Autodesk Inventor part; units mm, degrees
ref_plane "YZ Plane" through (0, 0, 0) normal (1, 0, 0) x (0, 1, 0)
ref_plane "XZ Plane" through (0, 0, 0) normal (0, 1, 0) x (-1, 0, 0)
ref_plane "XY Plane" through (0, 0, 0) normal (0, 0, 1) x (1, 0, 0)
sketch "スケッチ1" plane through (0, 0, 0) normal (0, 1, 0) x (-1, 0, 0)
  line L0 (0, 0) -> (-38, 0)
  line L1 (-38, 0) -> (-38, -48)
  line L2 (-38, -48) -> (0, -48)
  line L3 (0, -48) -> (0, 0)
  dimension "d0" = 48
  dimension "d1" = 38
extrude "押し出し1" add sketch "スケッチ1" along normal blind 46
sketch "スケッチ2" plane through (38, 0, -48) normal (0, 0, -1) x (-1, 0, 0)
  line L0 (3, 43) -> (59.072, 43)
  line L1 (59.072, 43) -> (59.072, 3)
  line L2 (59.072, 3) -> (3, 3)
  line L3 (3, 3) -> (3, 43)
  line L4 (0, 46) -> (38, 46)
  line L5 (0, 0) -> (38, 0)
  line L6 (0, 0) -> (0, 46)
  dimension "d4" = 40
  dimension "d6" = 3
  dimension "d7" = 3
extrude "押し出し2" cut sketch "スケッチ2" against normal blind 100
sketch "スケッチ3" plane through (0, 46, 0) normal (0, 1, 0) x (1, 0, 0)
  line L0 (38, 48) -> (0, 48)
  line L1 (38, 0) -> (38, 48)
  point P0 (0, 0)
  point P1 (17, 32)
  dimension "d10" = 16
  dimension "d11" = 21
hole "穴1" at (17, 46, -32) direction (0, -1, 0) diameter 22 end through all
sketch "スケッチ4" plane through (0, 46, 0) normal (0, 1, 0) x (1, 0, 0)
  line L0 (0, 0) -> (38, 0)
  line L1 (38, 0) -> (38, 48)
  point P0 (30.5, 4)
  point P1 (30.5, 31)
  point P2 (3.5, 4)
  point P3 (3.5, 31)
  point P4 (3.5, 4)
  dimension "d19" = 4
  dimension "d20" = 7.5
  dimension "d23" = 27
  dimension "d26" = 27
hole "穴2" at (30.5, 46, -4) at (30.5, 46, -31) at (3.5, 46, -31) at (3.5, 46, -4) direction (0, -1, 0) diameter 3.2 end through all
sketch "スケッチ6" plane through (38, 0, 0) normal (1, 0, 0) x (0, 0, -1)
  line L0 (0, 46) -> (48, 46)
  line L1 (0, 0) -> (0, 46)
  point P0 (10, 31)
  point P1 (32, 31)
  point P2 (10, 16)
  point P3 (32, 16)
  dimension "d45" = 15
  dimension "d46" = 10
  dimension "d49" = 22
  dimension "d52" = 15
fillet "フィレット1" radius 2 2 edges at (35, 3, -24) (35, 43, -24)
sketch "スケッチ8" plane through (35, 5, -48) normal (-1, 0, 0) x (0, 0, 1)
  line L0 (16, 11) -> (38, 11)
  line L1 (38, 11) -> (38, 26)
  line L2 (38, 26) -> (16, 26)
  line L3 (16, 26) -> (16, 11)
  line L4 (48, 36) -> (48, 0)
  line L5 (48, 41) -> (0, 41)
  point P0 (48, -5)
  dimension "d73" = 10
  dimension "d74" = 22
  dimension "d75" = 15
  dimension "d76" = 15
hole "穴5" at (35, 16, -10) at (35, 16, -32) at (35, 31, -32) at (35, 31, -10) direction (1, 0, 0) diameter 2.5 end through all
sketch "スケッチ9" plane through (0, 46, 0) normal (0, 1, 0) x (1, 0, 0)
  line L0 (0, 48) -> (33, 48)
  line L1 (14.5, 48) -> (19.5, 48)
  line L2 (19.5, 48) -> (19.5, 38.0378)
  line L3 (19.5, 38.0378) -> (14.5, 38.0378)
  line L4 (14.5, 38.0378) -> (14.5, 48)
  circle A0 centre (17, 32) radius 11
  point P0 (0, 0)
  point P1 (14.5, 42.7121)
  point P2 (19.5, 42.7121)
  dimension "d84" = 5
  dimension "d85" = 2.5
extrude "押し出し4" cut sketch "スケッチ9" against normal blind 3 contours L0 L2 A0 L4
properties part number "サーボモータ固定２軸"
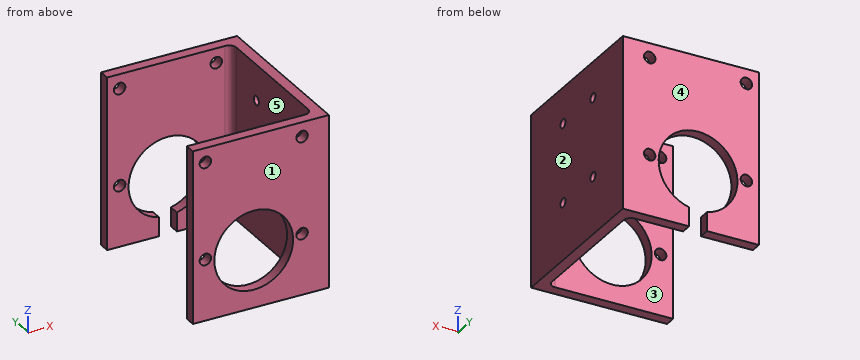
Source: CAD feature listing. Evaluate the final solid. Frame: model axes, mm. Face numbers are marked on the shaded views. A direction names the side the tool comes from. Coordinates: 2 decimals unless noted, no trailing zeros. Loops run counter-clockwise (first coordinate to the right, second up) from the corner with the lowest first, then second, coordinate; pieces in that order, holes last. Notation, with made-up numbers: M -35,-39 L -25,-39 A25 cw -25,-14 Z; hole C 81.25,71 d3. An arc over 180 degrees is marked long. Answer in a Markdown table with one row per item.
Q1. Ray query, probe 1 along Z at (x, y) = (30.5, 2.05); probe 2 along Y at (x, z) = (36, -10); probe 3 along Y at (x, z) = (13.5, -21). Return the intervals inside material, ascending. Write a range as from..to.
Answers below:
| item | result |
|---|---|
| probe 1 | z = -48..-32.6, -29.4..-5.6, -2.4..0 |
| probe 2 | y = 0..14.75, 17.25..29.75, 32.25..46 |
| probe 3 | y = 0..3, 43..46 |
Q2. First-contact query: pin 1 (2.5 mm diameter, centred on x = 30.5, z = -31, fed in from -Y); pin 2 (11 mm diameter, centred on y = 31.5, z = -21, fed in from -X). Flat tips, straight axial feed; report the tip coordinate or a pass-through.
Answers below:
| item | result |
|---|---|
| pin 1 | passes through |
| pin 2 | stops at x = 35 |
Q3. Section B-B on x = 3.5. Return the cut outline in (y, z), plus the area to 3 significant figures.
Answers below:
| item | result |
|---|---|
| outline | M 0,-48 L 3,-48 L 3,-32.6 L 0,-32.6 Z; M 0,-29.4 L 3,-29.4 L 3,-5.6 L 0,-5.6 Z; M 0,-2.4 L 3,-2.4 L 3,0 L 0,0 Z; M 43,-48 L 46,-48 L 46,-32.6 L 43,-32.6 Z; M 43,-29.4 L 46,-29.4 L 46,-5.6 L 43,-5.6 Z; M 43,-2.4 L 46,-2.4 L 46,0 L 43,0 Z |
| area | 250 mm^2 |
Q4. Draft query along Y for the marked faces 1, 2 and 3. Return one class per face: pulls with the +Y half, pulls with the -Y half, needs draft (parallel to the pull), parting line crosses it, or undercut.
Answers below:
| item | result |
|---|---|
| face 1 | pulls with the -Y half |
| face 2 | needs draft |
| face 3 | undercut |
Q5. Set-up query: the marked faces 4 and 5. Return all of +Z, -Z, +X, -X, +Y, -Y with unobstructed straight access to the full face (end or side cutting, diameter ignored); none if empty.
Answers below:
| item | result |
|---|---|
| face 4 | +Z, -Z, +X, -X, +Y |
| face 5 | +Z, -Z, -X |
Q6. Section C-C on y = 31. Return the cut outline in (x, z).
Answers below:
| item | result |
|---|---|
| outline | M 35,-48 L 38,-48 L 38,-33.25 L 35,-33.25 Z; M 35,-30.75 L 38,-30.75 L 38,-11.25 L 35,-11.25 Z; M 35,-8.75 L 38,-8.75 L 38,0 L 35,0 Z |
Q7. Section A-A on z = -10. Return the cut outline in (x, y), plus the area to 3 significant figures.
Answers below:
| item | result |
|---|---|
| outline | M 0,0 L 38,0 L 38,14.75 L 35,14.75 L 35,5 A2 cw 33,3 L 0,3 Z; M 0,43 L 33,43 A2 cw 35,41 L 35,32.25 L 38,32.25 L 38,46 L 0,46 Z; M 35,17.25 L 38,17.25 L 38,29.75 L 35,29.75 Z |
| area | 335 mm^2 |
Q8. Section D-D on x = 13.5. Return the cut outline in (y, z).
Answers below:
| item | result |
|---|---|
| outline | M 0,-48 L 3,-48 L 3,-42.43 L 0,-42.43 Z; M 0,-21.57 L 3,-21.57 L 3,0 L 0,0 Z; M 43,-48 L 46,-48 L 46,-42.43 L 43,-42.43 Z; M 43,-21.57 L 46,-21.57 L 46,0 L 43,0 Z |
